```python
from build123d import *


with BuildPart() as part:
    # Esquisse2 → Révolution1 (revolve)
    with BuildSketch(Plane.XY, mode=Mode.PRIVATE) as r_volution1_sk:
        with BuildLine():
            Line((7.95, 3.2), (7.95, 0))
            Line((7.95, 0), (10, 0))
            Line((10, 0), (10, 0.8))
            Line((10, 0.8), (11.9, 0.8))
            Line((11.9, 0.8), (11.9, 1.2))
            ThreePointArc((11.9, 1.2), (11.314213562, 2.614213562), (9.9, 3.2))
            Line((9.9, 3.2), (7.95, 3.2))
        make_face()
    r_volution1 = revolve(r_volution1_sk.sketch.rotate(Axis((0, 0, 0), (0, 1, 0)), 90), axis=Axis((0, 0, 0), (0, 1, 0)))

    # Symétrie1: Révolution1 across plane
    add(r_volution1.mirror(Plane.ZX))


solid = part.part
```
CAD build for the part. Positions are in the model's coordinates, mm. A direction names the side the tool comes from. Round coordinates to 2 decimals unless told otherwise and drop trailing zeros. Loops run counter-clockwise (first coordinate to the right, second up) from the corner with the lowest first, then second, coordinate; pieces in that order, holes last. Notation, with made-up numbers: M 43.5,-22 L 84.5,-22 A31 ccw 84.5,15 Z; hole C 37,52.5 d4. An arc over 180 degrees is marked long. Use a Markdown table: item, result. Add a question column.
(1) Cut at B-B (x = 0). Give the cut face in (y, z).
(2) Flat gauge pins, fed straight in: pin 1 (2 mm diameter, centred on x = -8.5, y = -1, fed in from +Z); pin 2 (1 mm diameter, centred on x = 6, y = -0.5, fed in from -Z). Where does each tip first touch, or does it go through?
(3) Which spindle directions (+Z, -Z, +X, -X, +Y, -Y) get a long thin tool onto all of the face, cutting with end or side? Do faces 4 (the face through (-8.043, -1.003, 8.771)), 5 (the face through (-10, 0.8, -3)). Say none if no direction does.
(4) Pull direction Y, two halves, no side cores. Call faces 1 (the face through (-8.11, 3.2, 0.05)), 2 (the face through (-8.11, -3.2, 0.05)), 3 (the face through (-10, -0.8, -3)): +Y half, -Y half, draft (parallel to the pull), parting line (faces both ways), or undercut.
(5) Drill centre lines: line 1 (X direction, y = 0.95, z = 0); line 2 (X direction, y = 0.75, z = 0); line 3 (Y direction, x = -8.5, z = 7). Where is each one in solid material? Low to high.
(6) Cut at C-C (y = -0.5). Give the cut face in (x, z), and give its area (3 significant figures).
(7) Cut at A-A (z = 0). Give the cut face in (x, y).
(8) Cut at D-D (y = -2.5). Give the cut face in (x, z).
Geometry says:
| question | item | result |
|---|---|---|
| 1 | outline | M -3.2,-9.9 A2 ccw -1.2,-11.9 L -0.8,-11.9 L -0.8,-10 L 0.8,-10 L 0.8,-11.9 L 1.2,-11.9 A2 ccw 3.2,-9.9 L 3.2,-7.95 L -3.2,-7.95 Z; M -3.2,7.95 L 3.2,7.95 L 3.2,9.9 A2 ccw 1.2,11.9 L 0.8,11.9 L 0.8,10 L -0.8,10 L -0.8,11.9 L -1.2,11.9 A2 ccw -3.2,9.9 Z |
| 2 | pin 1 | stops at z = 9.24 |
| 2 | pin 2 | stops at z = -10.5 |
| 3 | face 4 | +Y, -Y |
| 3 | face 5 | none |
| 4 | face 1 | +Y half |
| 4 | face 2 | -Y half |
| 4 | face 3 | undercut |
| 5 | line 1 | x = -11.9 to -7.95, 7.95 to 11.9 |
| 5 | line 2 | x = -10 to -7.95, 7.95 to 10 |
| 5 | line 3 | y = -2.86 to -0.8, 0.8 to 2.86 |
| 6 | outline | C 0,0 d20; hole C 0,0 d15.9 |
| 6 | area | 116 mm² |
| 7 | outline | M -11.9,-1.2 A2 ccw -9.9,-3.2 L -7.95,-3.2 L -7.95,3.2 L -9.9,3.2 A2 ccw -11.9,1.2 L -11.9,0.8 L -10,0.8 L -10,-0.8 L -11.9,-0.8 Z; M 7.95,-3.2 L 9.9,-3.2 A2 ccw 11.9,-1.2 L 11.9,-0.8 L 10,-0.8 L 10,0.8 L 11.9,0.8 L 11.9,1.2 A2 ccw 9.9,3.2 L 7.95,3.2 Z |
| 8 | outline | C 0,0 d22.84; hole C 0,0 d15.9 |
